from build123d import *

# Parameters (mm, degrees)
EXTRUDE_1_DEPTH = 6
SKETCH_2_R      = 2.5
EXTRUDE_2_DEPTH = 10


with BuildPart() as part:
    # 草圖1 → 伸長1 (new body)
    with BuildSketch(Plane.XY):
        with BuildLine():
            Line((-6, 40), (-6, 0))
            ThreePointArc((-6, 0), (0, -6), (6, 0))
            Line((6, 0), (6, 40))
            Line((6, 40), (-6, 40))
        make_face()
    extrude(amount=EXTRUDE_1_DEPTH)

    # 草圖2 → 伸長2 (add)
    with BuildSketch(Plane(origin=(0, 0, 0), x_dir=(-1, 0, 0), z_dir=(0, 0, -1))):
        with Locations(Location((0, 0, 0), (0, 0, 180))):
            Circle(SKETCH_2_R)
    extrude(amount=EXTRUDE_2_DEPTH)


solid = part.part
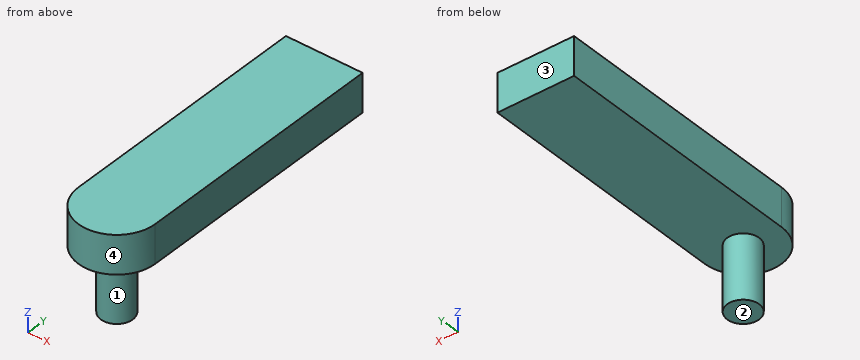
Here's how the part is built. I have some questions about the finished solid (model axes, mm). Face numbers are marked on the shaded views. Coordinates: 2 decimals unless noted, no trailing zeros. Write each loop counter-clockwise with the first axis right and the second up, starting at its lowest first coordinate (ties: lowest second). Pieces come first, ordered by that corner, then holes.
1) If we section it at D-D (y = 32.5): List the corners of the cut face in (x, z) for me.
Filled in:
outline: (-6, 0) - (6, 0) - (6, 6) - (-6, 6) - close
2) If we section it at A-A (y = 1.5): List the corners of the cut face in (x, z) for me.
Filled in:
outline: (-6, 0) - (-2, 0) - (-2, -10) - (2, -10) - (2, 0) - (6, 0) - (6, 6) - (-6, 6) - close
3) If I drill on line 1 (Z direction, x = 0, y = 11); line 2 (X direction, y = -1.5, z = -6); line 3 (Y direction, x = 5.25, z = 4.5), over which ranges is the centre line in solid material (lowest first)?
Filled in:
line 1: z = 0 to 6
line 2: x = -2 to 2
line 3: y = -2.9 to 40
4) Thinking about a two-plate mould opening in Y: for the marked faces 1, 2, 3 and 4, which applies, +Y half, -Y half, draft (parallel to the pull), parting line (faces both ways), or undercut?
Filled in:
face 1: parting line
face 2: draft
face 3: +Y half
face 4: -Y half
5) If we section it at C-C (z = 2.75): List the corners of the cut face in (x, y) for me, plus the area to 3 significant figures.
Filled in:
outline: (-6, 0) arc R6 ccw to (6, 0) - (6, 40) - (-6, 40) - close
area: 537 mm2
6) I'm going to push flat-ended pins straight in: pin 1 (6 mm diameter, centred on x = 2.5, y = 13.5, fed in from -Z); pin 2 (8 mm diameter, centred on y = 3.5, z = -7.5, fed in from -X); pin 3 (1 mm diameter, centred on y = 4, z = -4, fed in from -X); pin 4 (2 mm diameter, centred on x = 1.5, z = -6.5, fed in from +Y). Where does each tip first touch, or does it pass through?
Filled in:
pin 1: stops at z = 0
pin 2: stops at x = -2.5
pin 3: passes through
pin 4: stops at y = 2.45
7) If we section it at B-B (x = 0): List the corners of the cut face in (y, z) for me.
Filled in:
outline: (-6, 0) - (-2.5, 0) - (-2.5, -10) - (2.5, -10) - (2.5, 0) - (40, 0) - (40, 6) - (-6, 6) - close
